from build123d import *

# Parameters (mm, degrees)
BOX229_W         = 10
BOX229_H         = 25
BOX229_DEPTH     = 10
BOX228_W         = 10
BOX228_H         = 25
BOX228_DEPTH     = 10
SKETCH009_W      = 195
SKETCH009_H      = 105
SKETCH009_R      = 1.75
SKETCH009_W_2    = 165
SKETCH009_H_2    = 75
EXTRUDE009_DEPTH = 15
BOX223_W         = 11
BOX223_H         = 15
BOX223_DEPTH     = 65
BOX224_W         = 15
BOX224_H         = 15
BOX224_DEPTH     = 65
BOX225_W         = 15
BOX225_H         = 15
BOX225_DEPTH     = 65
BOX226_W         = 15
BOX226_H         = 15
BOX226_DEPTH     = 65
BOX227_W         = 15
BOX227_H         = 15
BOX227_DEPTH     = 65
BOX222_W         = 10
BOX222_H         = 15
BOX222_DEPTH     = 65
SKETCH013_R      = 2
EXTRUDE013_DEPTH = 30
BOX217_W         = 15
BOX217_H         = 15
BOX217_DEPTH     = 65
BOX218_W         = 15
BOX218_H         = 15
BOX218_DEPTH     = 65
BOX220_W         = 15
BOX220_H         = 15
BOX220_DEPTH     = 65
BOX216_W         = 15
BOX216_H         = 15
BOX216_DEPTH     = 65
BOX221_W         = 10
BOX221_H         = 23
BOX221_DEPTH     = 10
EXTRUDE012_DEPTH = 45.5
SKETCH014_R      = 1.5
EXTRUDE014_DEPTH = 30
SKETCH010_W      = 195
SKETCH010_H      = 105
SKETCH010_R      = 1.75
SKETCH010_R_2    = 1.25
SKETCH010_R_3    = 1.5
SKETCH010_W_2    = 165
SKETCH010_H_2    = 75
EXTRUDE010_DEPTH = 15


with BuildPart() as cube229:
    # Box229 → Box229 (new body)
    with BuildSketch(Plane(origin=(48, -69, 0), x_dir=(1, 0, 0), z_dir=(0, 0, 1))):
        with Locations((5, 12.5)):
            Rectangle(BOX229_W, BOX229_H)
    extrude(amount=BOX229_DEPTH)


with BuildPart() as ips_hold:
    # Box228 → Box228 (new body)
    with BuildSketch(Plane(origin=(-7, -69, 0), x_dir=(1, 0, 0), z_dir=(0, 0, 1))):
        with Locations((5, 12.5)):
            Rectangle(BOX228_W, BOX228_H)
    extrude(amount=BOX228_DEPTH)

    # Fusion132: union Cube229
    add(cube229.part)


with BuildPart() as ips_hold_1:
    # Fusion132 placement: moved
    add(ips_hold.part.moved(Location((0, 0, -62))))


with BuildPart() as sensor_base:
    # Sketch009 → Extrude009 (new body)
    with BuildSketch(Plane.XY):
        with Locations((60, -96)):
            Rectangle(SKETCH009_W, SKETCH009_H)
        with Locations((-30, -51)):
            Circle(SKETCH009_R, mode=Mode.SUBTRACT)
        with Locations((-30, -81)):
            Circle(SKETCH009_R, mode=Mode.SUBTRACT)
        with Locations((-30, -111)):
            Circle(SKETCH009_R, mode=Mode.SUBTRACT)
        with Locations((-30, -141)):
            Circle(SKETCH009_R, mode=Mode.SUBTRACT)
        with Locations((60, -141)):
            Circle(SKETCH009_R, mode=Mode.SUBTRACT)
        with Locations((150, -141)):
            Circle(SKETCH009_R, mode=Mode.SUBTRACT)
        with Locations((150, -111)):
            Circle(SKETCH009_R, mode=Mode.SUBTRACT)
        with Locations((150, -81)):
            Circle(SKETCH009_R, mode=Mode.SUBTRACT)
        with Locations((150, -51)):
            Circle(SKETCH009_R, mode=Mode.SUBTRACT)
        with Locations((60, -51)):
            Circle(SKETCH009_R, mode=Mode.SUBTRACT)
        with Locations((60, -96)):
            Rectangle(SKETCH009_W_2, SKETCH009_H_2, mode=Mode.SUBTRACT)
    extrude(amount=EXTRUDE009_DEPTH)


with BuildPart() as sensor_base_1:
    # Extrude009 placement: moved
    add(sensor_base.part.moved(Location((0, 0, -157))))


with BuildPart() as cube223:
    # Box223 → Box223 (new body)
    with BuildSketch(Plane(origin=(36, 0, -142), x_dir=(1, 0, 0), z_dir=(0, 0, 1))):
        with Locations((5.5, 7.5)):
            Rectangle(BOX223_W, BOX223_H)
    extrude(amount=BOX223_DEPTH)


with BuildPart() as cube224:
    # Box224 → Box224 (new body)
    with BuildSketch(Plane(origin=(93, 0, -142), x_dir=(1, 0, 0), z_dir=(0, 0, 1))):
        with Locations((7.5, 7.5)):
            Rectangle(BOX224_W, BOX224_H)
    extrude(amount=BOX224_DEPTH)


with BuildPart() as cube225:
    # Box225 → Box225 (new body)
    with BuildSketch(Plane(origin=(143, 15, -142), x_dir=(1, 0, 0), z_dir=(0, 0, 1))):
        with Locations((7.5, 7.5)):
            Rectangle(BOX225_W, BOX225_H)
    extrude(amount=BOX225_DEPTH)


with BuildPart() as cube226:
    # Box226 → Box226 (new body)
    with BuildSketch(Plane(origin=(-37, 45, -142), x_dir=(1, 0, 0), z_dir=(0, 0, 1))):
        with Locations((7.5, 7.5)):
            Rectangle(BOX226_W, BOX226_H)
    extrude(amount=BOX226_DEPTH)


with BuildPart() as cube227:
    # Box227 → Box227 (new body)
    with BuildSketch(Plane(origin=(143, 75, -142), x_dir=(1, 0, 0), z_dir=(0, 0, 1))):
        with Locations((7.5, 7.5)):
            Rectangle(BOX227_W, BOX227_H)
    extrude(amount=BOX227_DEPTH)


with BuildPart() as vertical_back:
    # Box222 → Box222 (new body)
    with BuildSketch(Plane(origin=(-4.5, 0, -142), x_dir=(1, 0, 0), z_dir=(0, 0, 1))):
        with Locations((5, 7.5)):
            Rectangle(BOX222_W, BOX222_H)
    extrude(amount=BOX222_DEPTH)

    # Fusion130: union Cube223, Cube224, Cube225, Cube226, Cube227
    add(cube223.part)
    add(cube224.part)
    add(cube225.part)
    add(cube226.part)
    add(cube227.part)


with BuildPart() as vertical_back_1:
    # Fusion130 placement: moved
    add(vertical_back.part.moved(Location((-0.5, -148.5, 0))))


with BuildPart() as obj1:
    # Sketch013 → Extrude013 (new body)
    with BuildSketch(Plane(origin=(0, 0, 0), x_dir=(-1, 0, 0), z_dir=(0, 1, 0))):
        with Locations((-29, -99.75)):
            Circle(SKETCH013_R)
        with Locations((15, -99.75)):
            Circle(SKETCH013_R)
        with Locations((15, -124.75)):
            Circle(SKETCH013_R)
        with Locations((-76, -105.5)):
            Circle(SKETCH013_R)
        with Locations((-119.5, -105.5)):
            Circle(SKETCH013_R)
        with Locations((-97.75, -67.827895)):
            Circle(SKETCH013_R)
    extrude(amount=-EXTRUDE013_DEPTH)


with BuildPart() as obj1_1:
    # Extrude013 placement: moved
    add(obj1.part.moved(Location((0, -36, 0))))


with BuildPart() as cube217:
    # Box217 → Box217 (new body)
    with BuildSketch(Plane(origin=(22, 0, -142), x_dir=(1, 0, 0), z_dir=(0, 0, 1))):
        with Locations((7.5, 7.5)):
            Rectangle(BOX217_W, BOX217_H)
    extrude(amount=BOX217_DEPTH)


with BuildPart() as cube218:
    # Box218 → Box218 (new body)
    with BuildSketch(Plane(origin=(69, 0, -142), x_dir=(1, 0, 0), z_dir=(0, 0, 1))):
        with Locations((7.5, 7.5)):
            Rectangle(BOX218_W, BOX218_H)
    extrude(amount=BOX218_DEPTH)


with BuildPart() as cube220:
    # Box220 → Box220 (new body)
    with BuildSketch(Plane(origin=(113, 0, -142), x_dir=(1, 0, 0), z_dir=(0, 0, 1))):
        with Locations((7.5, 7.5)):
            Rectangle(BOX220_W, BOX220_H)
    extrude(amount=BOX220_DEPTH)


with BuildPart() as cut017:
    # Box216 → Box216 (new body)
    with BuildSketch(Plane(origin=(-22, 0, -142), x_dir=(1, 0, 0), z_dir=(0, 0, 1))):
        with Locations((7.5, 7.5)):
            Rectangle(BOX216_W, BOX216_H)
    extrude(amount=BOX216_DEPTH)

    # Fusion129: union Cube217, Cube218, Cube220
    add(cube217.part)
    add(cube218.part)
    add(cube220.part)


with BuildPart() as cut017_1:
    # Fusion129 placement: moved
    add(cut017.part.moved(Location((-0.5, -58.5, 0))))

    # Cut017: cut obj1
    add(obj1_1.part, mode=Mode.SUBTRACT)


with BuildPart() as cube221:
    # Box221 → Box221 (new body)
    with BuildSketch(Plane(origin=(27.5, -21, -114.5), x_dir=(1, 0, 0), z_dir=(0, 0, 1))):
        with Locations((5, 11.5)):
            Rectangle(BOX221_W, BOX221_H)
    extrude(amount=BOX221_DEPTH)


with BuildPart() as cut016:
    # Sketch012 → Extrude012 (new body)
    with BuildSketch(Plane(origin=(0, 0, 0), x_dir=(-1, 0, 0), z_dir=(0, 1, 0))):
        Polygon((-80.36, -110.5), (-68.5, -110.5), (-68.5, -114.5), (-76.36, -114.5), (-76.36, -127.5), (-68.56, -127.5), (-68.56, -131.5), (-80.36, -131.5), align=None)
        Polygon((-36.5, -127.5), (-36.5, -131.5), (-23.5, -131.5), (-23.5, -110.5), (-36.5, -110.5), (-36.5, -114.5), (-27.5, -114.5), (-27.5, -127.5), align=None)
    extrude(amount=-EXTRUDE012_DEPTH)


with BuildPart() as cut016_1:
    # Extrude012 placement: moved
    add(cut016.part.moved(Location((0, 2, 0))))

    # Cut016: cut Cube221
    add(cube221.part, mode=Mode.SUBTRACT)


with BuildPart() as cut016_2:
    # Cut016 placement: moved
    add(cut016_1.part.moved(Location((47.14, -60.5, 0))))


with BuildPart() as extrude014:
    # Sketch014 → Extrude014 (new body)
    with BuildSketch(Plane(origin=(0, 0, 0), x_dir=(0, -1, 0), z_dir=(-1, 0, 0))):
        with Locations((114.65, -69.85)):
            Circle(SKETCH014_R)
        with Locations((127.35, -69.85)):
            Circle(SKETCH014_R)
    extrude(amount=EXTRUDE014_DEPTH)


with BuildPart() as extrude014_1:
    # Extrude014 placement: moved
    add(extrude014.part.moved(Location((-15, 0, 0))))


with BuildPart() as sensor_hold:
    # Sketch010 → Extrude010 (new body)
    with BuildSketch(Plane.XY):
        with Locations((60, -96)):
            Rectangle(SKETCH010_W, SKETCH010_H)
        with Locations((-30, -51)):
            Circle(SKETCH010_R, mode=Mode.SUBTRACT)
        with Locations((-30, -81)):
            Circle(SKETCH010_R, mode=Mode.SUBTRACT)
        with Locations((-30, -111)):
            Circle(SKETCH010_R, mode=Mode.SUBTRACT)
        with Locations((-30, -141)):
            Circle(SKETCH010_R, mode=Mode.SUBTRACT)
        with Locations((60, -141)):
            Circle(SKETCH010_R, mode=Mode.SUBTRACT)
        with Locations((150, -141)):
            Circle(SKETCH010_R, mode=Mode.SUBTRACT)
        with Locations((150, -111)):
            Circle(SKETCH010_R, mode=Mode.SUBTRACT)
        with Locations((150, -81)):
            Circle(SKETCH010_R, mode=Mode.SUBTRACT)
        with Locations((150, -51)):
            Circle(SKETCH010_R, mode=Mode.SUBTRACT)
        with Locations((60, -51)):
            Circle(SKETCH010_R, mode=Mode.SUBTRACT)
        with Locations((7.5, -51)):
            Circle(SKETCH010_R_2, mode=Mode.SUBTRACT)
        with Locations((-9.75, -141)):
            Circle(SKETCH010_R_3, mode=Mode.SUBTRACT)
        with Locations((10.55, -141)):
            Circle(SKETCH010_R_3, mode=Mode.SUBTRACT)
        with Locations((30.8, -141)):
            Circle(SKETCH010_R_3, mode=Mode.SUBTRACT)
        with Locations((51.1, -141)):
            Circle(SKETCH010_R_3, mode=Mode.SUBTRACT)
        with Locations((71.4, -141)):
            Circle(SKETCH010_R_3, mode=Mode.SUBTRACT)
        with Locations((129.4, -141)):
            Circle(SKETCH010_R_3, mode=Mode.SUBTRACT)
        with Locations((60, -96)):
            Rectangle(SKETCH010_W_2, SKETCH010_H_2, mode=Mode.SUBTRACT)
    extrude(amount=EXTRUDE010_DEPTH)


with BuildPart() as sensor_hold_1:
    # Extrude010 placement: moved
    add(sensor_hold.part.moved(Location((0, 0, -77))))

    # Cut018: cut Extrude014
    add(extrude014_1.part, mode=Mode.SUBTRACT)

    # Fusion131: union Sensor_base, Vertical_back, Cut017, Cut016
    add(sensor_base_1.part)
    add(vertical_back_1.part)
    add(cut017_1.part)
    add(cut016_2.part)

    # Fusion133: union ips_hold
    add(ips_hold_1.part)


solid = sensor_hold_1.part
Design review of the part built by this model. Coordinates are the model's own, in mm. A direction names the side the tool comes from. Coordinates: 2 decimals unless noted, no trailing zeros. Order: outer loops, then holes, each group sorted by start corner. A loop starts at its lowest first (then second) coordinate and runs counter-clockwise, first axis right, second up. Notation, with made-up numbers: (75, 50.5) -> (106, 50.5) arc R19 ccw to (106, 85.5) -> close; hole circle Ø2 at (45, 29). An arc over 180 degrees is marked (long way). Use one line per item in the form item = value. Start each with the question number.
(1) Add section A-A on x = 55.5. State the section outline as (y, z) points, plus the area to 3 significant figures.
(2) Add section D-D on z = -117. Give the number of separate pieces and of enclosed holes in the cut face, plus the area to 3 significant figures.
(3) Add section B-B on y = -99. State the section outline as (x, z) points.
(4) Add section C-C on x = -15. State the section outline as (y, z) points.
(5) Insertion check: pin 1 (16.5 mm diameter, centred on x = 96, y = -52, fed in from +Z); pin 2 (13 mm diameter, centred on x = 120, z = -117.5, fed in from -Y); pin 3 (1.5 mm diameter, centred on y = -137, z = -110, fed in from -X). Each pin has a flat end and moves straight along its axis. Give the tip position at first contact, or say it passes through.
(6) For faces 4 (the flat face through (150, -96, -142)), 5 (the flat face through (48, -57, -57)), 6 (the flat face through (142, -51, -142)), 7 (the flat face through (36.5, -51, -110)), 8 (the flat face through (-22.5, -93, -106)), list the 3-axis set-ups (+Z, -Z, +X, -X, +Y, -Y) from which the entire face can be reached by the end or side of a thin tool; tool diameter is ignored.
(7) For probe 1 along X at (y, z) = (-81, -149.5); probe 2 along X at (y, z) = (-60.5, -127); probe 3 along Y at (x, z) = (150, -70), list the stretches that pass through material, from the lowest coordinate up.
(8) The part is to be moulded in two halves that separate along X. For faces 1 (the flat face through (21.5, -51, -110)), 2 (the flat face through (58, -57, -57)), 3 (the flat face through (-30, -66, -142)), say which applies: +X half, -X half, draft (parallel to the pull), parting line (faces both ways), or undercut.
Answer block:
q1.outline = (-148.5, -157) -> (-133.5, -157) -> (-133.5, -142) -> (-148.5, -142) -> close; (-148.5, -77) -> (-133.5, -77) -> (-133.5, -62) -> (-148.5, -62) -> close; (-69, -62) -> (-58.5, -62) -> (-58.5, -77) -> (-43.5, -77) -> (-43.5, -62) -> (-44, -62) -> (-44, -52) -> (-69, -52) -> close; (-58.5, -157) -> (-43.5, -157) -> (-43.5, -142) -> (-58.5, -142) -> close
q1.area = 1,150 mm²
q2.separate_pieces = 10
q2.enclosed_holes = 0
q2.area = 2,480 mm²
q3.outline = (-37.5, -157) -> (-22.5, -157) -> (-22.5, -62) -> (-37.5, -62) -> close; (70.64, -131.5) -> (83.64, -131.5) -> (83.64, -127.5) -> (74.64, -127.5) -> (74.64, -114.5) -> (83.64, -114.5) -> (83.64, -110.5) -> (70.64, -110.5) -> close; (115.64, -114.5) -> (123.5, -114.5) -> (123.5, -127.5) -> (115.7, -127.5) -> (115.7, -131.5) -> (127.5, -131.5) -> (127.5, -110.5) -> (115.64, -110.5) -> close; (142.5, -157) -> (157.5, -157) -> (157.5, -142) -> (142.5, -142) -> close; (142.5, -77) -> (157.5, -77) -> (157.5, -62) -> (142.5, -62) -> close
q4.outline = (-148.5, -157) -> (-133.5, -157) -> (-133.5, -142) -> (-148.5, -142) -> close; (-148.5, -77) -> (-133.5, -77) -> (-133.5, -62) -> (-148.5, -62) -> close; (-58.5, -157) -> (-43.5, -157) -> (-43.5, -126.75) -> (-58.5, -126.75) -> close; (-58.5, -122.75) -> (-43.5, -122.75) -> (-43.5, -101.75) -> (-58.5, -101.75) -> close; (-58.5, -97.75) -> (-43.5, -97.75) -> (-43.5, -62) -> (-58.5, -62) -> close
q5.pin_1 = -62
q5.pin_2 = -104
q5.pin_3 = -5
q6.face_4 = +X
q6.face_5 = +Z, +Y, -Y
q6.face_6 = +X, +Y
q6.face_7 = +Y
q6.face_8 = +Z, -Z
q7.probe_1 = -37.5 to -31.75, -28.25 to -22.5, 142.5 to 148.25, 151.75 to 157.5
q7.probe_2 = 70.64 to 74.64, 123.5 to 127.5, 142.5 to 157.5
q7.probe_3 = -148.5 to -142.75, -139.25 to -112.75, -109.25 to -82.75, -79.25 to -52.75, -49.25 to -43.5
q8.face_1 = undercut
q8.face_2 = +X half
q8.face_3 = draft
